Geometry: final body of the model. Coordinates: model frame, mm. Face numbers are marked on the shaded views. A direction names the side the tool comes from. Round coordinates to 2 decimals unless told otherwise and drop trailing zeros. Order: outer loops, then holes, each group sorted by start corner. A loop starts at its lowest first (then second) coordinate and runs counter-clockwise, first axis right, second up. Notation, with made-up numbers: M 82,3 L 87,3 A23 ccw 87,14 Z; hole C 61.5,0 d3. An arc over 180 degrees is marked long. Put each result on its own line as item: value. Start each with the question number.
1) Material intervals for probe 1 along Z at (x, y) = (103.5, 38); probe 2 along Y at (x, z) = (-19.5, -36.5); probe 3 along Y at (x, z) = (163.5, -17), sorted ascending. Write a range as [from, to].
2) Draft query along Z for the marked faces 4, 5 and 6. Return one class per face: pulls with the +Z half, pulls with the -Z half, needs draft (parallel to the pull), parting line crosses it, or undercut.
3) Section A-A, the plane x = -20.5. Return loops of the section in (y, z).
4) Access query for the marked faces 1, 2 and 3. Directions: +Z, -Z, +X, -X, +Y, -Y. A direction counts if a zero-diameter tool reaches every point of the face in a straight line with its end or side. Return the directions, or none.
5) Section B-B, the plane z = -31. Return loops of the section in (x, y).
6) First-contact query: P1, Ø4, axis at y = 30.5, z = -2, coming from the +X side; P2, Ø5, axis at x = 181, z = -2.5, coming from the +Y side; P3, Ø2, axis at x = 105, z = -7.5, coming from the +Y side. Flat tips, straight axial feed; report the tip coordinate or a pass-through.
from build123d import *

# Parameters (mm, degrees)
SKETCH1_W           = 190.5
SKETCH1_H           = 40.64
BOSS_EXTRUDE1_DEPTH = 50.8
SKETCH2_W           = 33.8328
SKETCH2_H           = 53.486117269
CUT_EXTRUDE1_DEPTH  = 202.302010919
BOSS_EXTRUDE2_REACH = 191.307
SKETCH4_W           = 196.307587048
SKETCH4_H           = 33.8328
SKETCH6_W           = 25.4
SKETCH6_H           = 50.8
CUT_EXTRUDE3_DEPTH  = 202.302010919
FILLET1_R           = 3.81
SKETCH7_W           = 25.4
SKETCH7_H           = 40.64
CUT_EXTRUDE4_DEPTH  = 5.08
SKETCH8_W           = 40.64
SKETCH8_H           = 50.8
BOSS_EXTRUDE3_DEPTH = 37.592
FILLET2_R           = 2.54
SKETCH9_W           = 37.592
SKETCH9_H           = 38.1
CUT_EXTRUDE5_DEPTH  = 202.302011039


with BuildPart() as part:
    # Sketch1 → Boss-Extrude1 (new body)
    with BuildSketch(Plane(origin=(0, 0, 0), x_dir=(1, 0, 0), z_dir=(0, 1, 0))):
        with Locations((95.25, 20.32)):
            Rectangle(SKETCH1_W, SKETCH1_H)
    extrude(amount=BOSS_EXTRUDE1_DEPTH)

    # Sketch2 → Cut-Extrude1 (cut, through all)
    with BuildSketch(Plane(origin=(190.5, 0, 0), x_dir=(0, 0, -1), z_dir=(1, 0, 0))):
        with Locations((20.32, 30.146658634)):
            Rectangle(SKETCH2_W, SKETCH2_H)
    extrude(amount=-CUT_EXTRUDE1_DEPTH, mode=Mode.SUBTRACT)

    # Boss-Extrude2: up to this face of the body (flat: up to its plane)
    boss_extrude2_end = Plane(part.part.faces().sort_by_distance((95.25, 3.4036, -20.32))[0])
    # Sketch4 → Boss-Extrude2 (add, up to the picked face)
    with BuildSketch(Plane(origin=(11.902272211, 47.838714674, 0), x_dir=(0.9704158808316984, -0.24143947115092654, 0), z_dir=(0.2414394711509265, 0.9704158808316983, 0)), mode=Mode.PRIVATE) as boss_extrude2_sk1:
        with Locations((85.88866839, 20.32)):
            Rectangle(SKETCH4_W, SKETCH4_H)
    boss_extrude2_tool1 = split(extrude(boss_extrude2_sk1.sketch, amount=-BOSS_EXTRUDE2_REACH, mode=Mode.PRIVATE), bisect_by=boss_extrude2_end, keep=Keep.BOTH, mode=Mode.PRIVATE)
    add(boss_extrude2_tool1.solids().sort_by(Axis((95.25, 27.1018, -20.32), (-0.2414394711509265, -0.9704158808316983, 0)))[0])

    # Sketch6 → Cut-Extrude3 (cut, through all)
    with BuildSketch(Plane.XY):
        with Locations((-12.7, 25.4)):
            Rectangle(SKETCH6_W, SKETCH6_H)
    extrude(amount=-CUT_EXTRUDE3_DEPTH, mode=Mode.SUBTRACT)

    # Fillet1
    fillet1_edges = [part.edges().sort_by_distance(p)[0] for p in [
        (95.25, 27.1018, -3.4036),
        (95.25, 27.1018, -37.2364),
    ]]
    fillet(fillet1_edges, radius=FILLET1_R)

    # Sketch7 → Cut-Extrude4 (cut)
    with BuildSketch(Plane.XY):
        with Locations((177.8, 30.48)):
            Rectangle(SKETCH7_W, SKETCH7_H)
    extrude(amount=-CUT_EXTRUDE4_DEPTH, mode=Mode.SUBTRACT)

    # Sketch8 → Boss-Extrude3 (add)
    with BuildSketch(Plane.ZY):
        with Locations((-20.32, 25.4)):
            Rectangle(SKETCH8_W, SKETCH8_H)
    extrude(amount=BOSS_EXTRUDE3_DEPTH)

    # Fillet2
    fillet2_edges = [part.edges().sort_by_distance(p)[0] for p in [
        (165.1, 10.16, -2.54),
    ]]
    fillet(fillet2_edges, radius=FILLET2_R)

    # Sketch9 → Cut-Extrude5 (cut, through all)
    with BuildSketch(Plane.XY):
        with Locations((-18.796, 25.4)):
            Rectangle(SKETCH9_W, SKETCH9_H)
    extrude(amount=-CUT_EXTRUDE5_DEPTH, mode=Mode.SUBTRACT)


solid = part.part
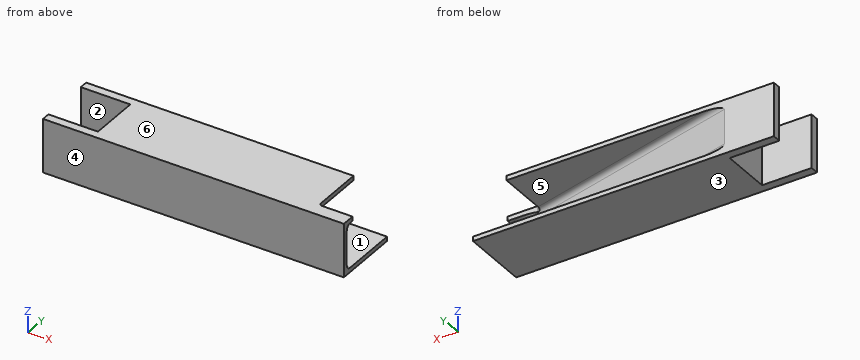
Result sheet:
1. probe 1: z = [-40.64, -37.24], [-3.4, 0]
1. probe 2: y = [0, 6.35], [44.45, 50.8]
1. probe 3: y = [0, 10.12]
2. face 4: needs draft
2. face 5: undercut
2. face 6: pulls with the +Z half
3. outline: M 0,-40.64 L 6.35,-40.64 L 6.35,0 L 0,0 Z; M 44.45,-40.64 L 50.8,-40.64 L 50.8,0 L 44.45,0 Z
4. face 1: +X, +Y
4. face 2: +Z, -Z, -X
4. face 3: -Z, +X, -X, +Y, -Y
5. outline: M -37.59,0 L 190.5,0 L 190.5,3.4 L 0,50.8 L -37.59,50.8 L -37.59,44.45 L 0,44.45 L 0,6.35 L -37.59,6.35 Z
6. P1: stops at x = 165.1
6. P2: stops at y = 10.16
6. P3: stops at y = 24.92
